Check sheet for the modelled part. Datum: model origin and axes. Units: mm. A direction names the side the tool comes from. Give positions to 0.01 mm unless a question says otherwise; leave off trailing zeros. Write each loop counter-clockwise with the first axis right and the second up, starting at its lowest first coordinate (ties: lowest second). Pieces come first, ordered by that corner, then holes. Notation, with made-up numbers: M 55.25,80 L 89.25,80 A24 cw 89.25,99 Z; hole C -32,74.5 d8. An arc over 180 degrees is marked long. Use CSV: the item, a comma, the result in double quotes. Start each with the question number.
1. Cross-section at C-C, the plane y = 0. Enter the section's corners in (x, z).
2. Scan lines: line 1 (X direction, y = -30.6, z = -26.5); line 2 (X direction, y = -29, z = 26); line 3 (Y direction, x = 28, z = -14.5). Record each from-to range of solid material in increasing order.
3. Depth check by flat-ended pin: P1, Ø2, axis at y = -17.5, z = -11, coming from the -X side; P2, Ø24.5, axis at y = 4.5, z = 0, coming from the -X side; P3, Ø20, axis at x = 26, z = 12.5, coming from the +Y side; P4, Ø13.5, axis at y = 0, z = 0, coming from the -X side. Enter the tip coordinate at first touch or a pass-through.
4. Cross-section at B-B, the plane z = 0. Enter the section's corners in (x, y), and give its area (3 significant figures).
5. Cross-section at D-D, the plane x = 34.5. Enter the section's corners in (y, z).
6. Cross-section at A-A, the plane x = 13.5. Enter the section's corners in (y, z), and give its area (3 significant figures).
7. Mould release check, pull along X, two halves, no side actions. Record for faces 1 (the face through (0, -4, 11)), 2 (the face through (10.88, -2.6, 8.25)), 3 (the face through (21, -30.2, 23.9)): +X half, -X half, draft (parallel to the pull), parting line (faces both ways), or undercut.
8. Access from +Z, -Z, +X, -X, +Y, -Y to the whole of each face (thin tool, end or side, straight path). Record for faces 4 (the face through (3.549, -3.349, 10.635)), 5 (the face through (18, -23, 1.5)), 6 (the face through (18, -23, -1.5)), 7 (the face through (14.653, -7, -7)).
from build123d import *

# Parameters (mm, degrees)
BOSS_EXTRUDE1_START = -7
BOSS_EXTRUDE1_DEPTH = 7
SKETCH6_W           = 63
SKETCH6_H           = 5
BOSS_EXTRUDE2_DEPTH = 25
SKETCH7_R           = 2.6
CUT_EXTRUDE1_DEPTH  = 73.836579806
BOSS_EXTRUDE3_DEPTH = 1.5


with BuildPart() as part:
    # Sketch4 → Revolve1 (revolve)
    with BuildSketch(Plane.XY, mode=Mode.PRIVATE) as revolve1_sk:
        Polygon((0, 11.15), (7, 11.15), (7, 8.65), (14.653434377, 8.65), (14.653434377, 24.65), (7.653434377, 24.65), (0, 16.15), align=None)
    revolve(revolve1_sk.sketch.rotate(Axis((0, 0, 0), (1, 0, 0)), 90), axis=Axis((0, 0, 0), (1, 0, 0)))

    # Sketch5 → Boss-Extrude1 (add)
    with BuildSketch(Plane(origin=(14.653434377, 0, 0), x_dir=(0, 0, -1), z_dir=(1, 0, 0)).offset(BOSS_EXTRUDE1_START)):
        with BuildLine():
            Line((-31.5, -32.7), (31.5, -32.7))
            Line((31.5, -32.7), (31.5, -27.7))
            Line((31.5, -27.7), (24.048586045, 5.411839727))
            ThreePointArc((24.048586045, 5.411839727), (0, -24.65), (-24.048586045, 5.411839727))
            Line((-24.048586045, 5.411839727), (-31.5, -27.7))
            Line((-31.5, -27.7), (-31.5, -32.7))
        make_face()
    extrude(amount=BOSS_EXTRUDE1_DEPTH)

    # Sketch6 → Boss-Extrude2 (add)
    with BuildSketch(Plane(origin=(14.653434377, 0, 0), x_dir=(0, 0, -1), z_dir=(1, 0, 0))):
        with Locations((0, -30.2)):
            Rectangle(SKETCH6_W, SKETCH6_H)
    extrude(amount=BOSS_EXTRUDE2_DEPTH)

    # Sketch7 → Cut-Extrude1 (cut, through all)
    with BuildSketch(Plane(origin=(0, -27.7, 0), x_dir=(1, 0, 0), z_dir=(0, 1, 0))):
        with Locations(Location((20.903434377, 26.5, 0), (0, 0, 270))):
            Circle(SKETCH7_R)
        with Locations(Location((33.403434377, 26.5, 0), (0, 0, 270))):
            Circle(SKETCH7_R)
        with Locations(Location((33.403434377, -26.5, 0), (0, 0, 270))):
            Circle(SKETCH7_R)
        with Locations(Location((20.903434377, -26.5, 0), (0, 0, 270))):
            Circle(SKETCH7_R)
    extrude(amount=-CUT_EXTRUDE1_DEPTH, mode=Mode.SUBTRACT)

    # Sketch8 → Boss-Extrude3 (add, symmetric)
    with BuildSketch(Plane.XY):
        Polygon((26.653434377, -27.7), (14.653434377, -12.7), (14.653434377, -27.7), align=None)
    extrude(amount=BOSS_EXTRUDE3_DEPTH, both=True)


solid = part.part
Worked answers:
1,outline,"M 0,-16.15 L 7.65,-24.65 L 7.65,-25.27 L 14.65,-25.27 L 14.65,-8.65 L 7,-8.65 L 7,-11.15 L 0,-11.15 Z; M 0,11.15 L 7,11.15 L 7,8.65 L 14.65,8.65 L 14.65,25.27 L 7.65,25.27 L 7.65,24.65 L 0,16.15 Z"
2,line 1,"x = 7.65 to 18.3, 23.5 to 30.8, 36 to 39.65"
2,line 2,"x = 7.65 to 18.35, 23.45 to 30.85, 35.95 to 39.65"
2,line 3,"y = -32.7 to -27.7"
3,P1,"stops at x = 3.17"
3,P2,"stops at x = 0"
3,P3,"stops at y = -27.7"
3,P4,"passes through"
4,outline,"M 0,-16.15 L 7.65,-24.65 L 7.65,-32.7 L 39.65,-32.7 L 39.65,-27.7 L 26.65,-27.7 L 14.65,-12.7 L 14.65,-8.65 L 7,-8.65 L 7,-11.15 L 0,-11.15 Z; M 0,11.15 L 7,11.15 L 7,8.65 L 14.65,8.65 L 14.65,24.65 L 7.65,24.65 L 0,16.15 Z"
4,area,"640 mm^2"
5,outline,"M -32.7,-31.5 L -27.7,-31.5 L -27.7,-28.86 L -32.7,-28.86 Z; M -32.7,-24.14 L -27.7,-24.14 L -27.7,24.14 L -32.7,24.14 Z; M -32.7,28.86 L -27.7,28.86 L -27.7,31.5 L -32.7,31.5 Z"
6,outline,"M -32.7,-31.5 L -27.7,-31.5 L 5.41,-24.05 A24.65 ccw 5.41,24.05 L -27.7,31.5 L -32.7,31.5 Z; hole C 0,0 d17.3"
6,area,"2,610 mm^2"
7,face 1,"-X half"
7,face 2,"draft"
7,face 3,"undercut"
8,face 4,"-X"
8,face 5,"+Z, +X, +Y"
8,face 6,"-Z, +X, +Y"
8,face 7,"+X, +Y"
